The listing builds one solid part. Answer for the finished solid, in the listing's coordinates (mm). Face numbers are marked on the shaded views. A direction names the side the tool comes from. Give positions to 0.01 mm unless a question says otherwise; leave off trailing zeros. Write each loop counter-clockwise with the first axis right and the second up, starting at its lowest first coordinate (ties: lowest second). Pieces come first, ordered by that corner, then holes. Notation, with made-up numbers: (81.25, 49) - (89.25, 49) arc R21 cw to (89.25, 76) - close; hole circle Ø5 at (35.25, 86). An arc over 180 degrees is marked (long way). Return JSON: item names as keys, results as strings.
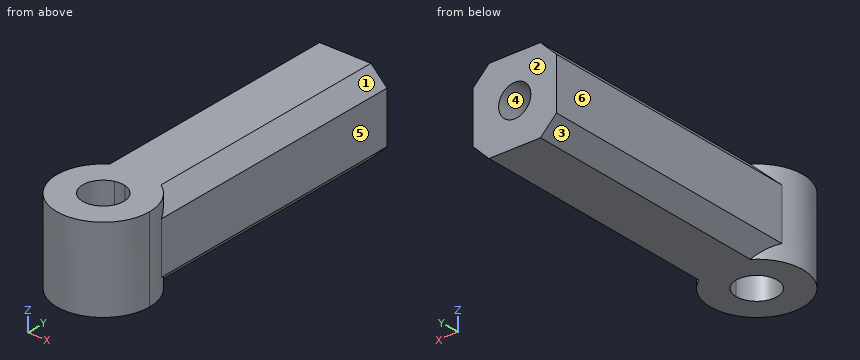
from build123d import *

# Parameters (mm, degrees)
F3_DEPTH = 6.5
F4_SIZE  = 1.25
F5_R     = 1.25
F6_DEPTH = 20


with BuildPart() as f3:
    # F2 (on Top) → F3 (new body)
    with BuildSketch(Plane.XY):
        with BuildLine():
            ThreePointArc((-3.25, 1.5483862567), (0, 3.6), (3.25, 1.5483862567))
            Line((3.25, 1.5483862567), (3.25, 22.5483862567))
            Line((3.25, 22.5483862567), (-3.25, 22.5483862567))
            Line((-3.25, 22.5483862567), (-3.25, 1.5483862567))
        make_face()
        with BuildLine():
            ThreePointArc((-0.4031128874, 1.5483862567), (0, 1.6), (0.4031128874, 1.5483862567))
            Line((0.4031128874, 1.5483862567), (3.25, 1.5483862567))
            ThreePointArc((3.25, 1.5483862567), (0, 3.6), (-3.25, 1.5483862567))
            Line((-3.25, 1.5483862567), (-0.4031128874, 1.5483862567))
        make_face()
        with BuildLine():
            ThreePointArc((0.4031128874, 1.5483862567), (1.2658950628, 0.9785242409), (1.6, 0))
            ThreePointArc((1.6, 0), (-0.9785242409, -1.2658950628), (-0.4031128874, 1.5483862567))
            Line((-0.4031128874, 1.5483862567), (-3.25, 1.5483862567))
            ThreePointArc((-3.25, 1.5483862567), (-0.7937253933, -3.5114099732), (3.6, 0))
            ThreePointArc((3.6, 0), (3.5114099732, 0.7937253933), (3.25, 1.5483862567))
            Line((3.25, 1.5483862567), (0.4031128874, 1.5483862567))
        make_face()
    extrude(amount=F3_DEPTH)

    # F4
    f4_edges = [f3.edges().sort_by_distance(p)[0] for p in [
        (3.25, 12.048386, 6.5),
        (-3.25, 12.048386, 6.5),
        (3.25, 12.048386, 0),
        (-3.25, 12.048386, 0),
    ]]
    chamfer(f4_edges, length=F4_SIZE)

    # F5 (on face) → F6 (cut)
    with BuildSketch(Plane(origin=(0, 22.5483862567, 0), x_dir=(-1, 0, 0), z_dir=(0, 1, 0))):
        with Locations((0, 3.25)):
            Circle(F5_R)
    extrude(amount=-F6_DEPTH, mode=Mode.SUBTRACT)


solid = f3.part
Item 1: Consider L1, parallel to Z at x = 0, y = 10; L2, parallel to Y at x = 0, z = 1.5; L3, parallel to Y at x = 0, z = 3.25. Determine where each line is inside the solid, lowest interval first.
Answer below:
{"L1": "z = 0 to 2, 4.5 to 6.5", "L2": "y = -3.6 to -1.6, 1.6 to 22.55", "L3": "y = -3.6 to -1.6, 1.6 to 2.55"}
Item 2: Flat-ended cylindrical pins translate along their axes: P1, Ø1, axis at y = -1, z = 3.5, coming from the -X side; P2, Ø1.2, axis at y = 17, z = 2.5, coming from the -X side; P3, Ø2, axis at x = -1.5, z = 3, coming from the -Y side. Find the tip coordinate at first contact, or state that the pin passes through.
Answer below:
{"P1": "stops at x = -3.57", "P2": "stops at x = -3.25", "P3": "stops at y = -3.57"}
Item 3: For the marked faces 1, 2 and 3, determine the directions among +Z, -Z, +X, -X, +Y, -Y from which every point of the face is accessible in a straight line to the end or side of a thin tool.
Answer below:
{"face 1": "+Z, +X, +Y", "face 2": "+Z, -Z, +X, -X, +Y", "face 3": "-Z, -X, +Y"}
Item 4: A cutting plane is placed at B-B on z = 3.25. Determine the outline of the cut face in (x, y), then the cut area to 3 significant figures.
Answer below:
{"outline": "(-3.25, 1.55) arc R3.6 ccw (long way) to (3.25, 1.55) - (3.25, 22.55) - (1.25, 22.55) - (1.25, 2.55) - (-1.25, 2.55) - (-1.25, 22.55) - (-3.25, 22.55) - close; hole circle Ø3.2 at (0, 0)", "area": "110 mm²"}
Item 5: The mould has two halves that part along X. Classify the marked faces 4, 5 and 6: +X half, -X half, draft (parallel to the pull), parting line (faces both ways), or undercut.
Answer below:
{"face 4": "undercut", "face 5": "+X half", "face 6": "-X half"}
Item 6: A cutting plane is placed at C-C on y = 6. Determine the outline of the cut face in (x, z), then the cut area to 3 significant figures.
Answer below:
{"outline": "(-3.25, 1.25) - (-2, 0) - (2, 0) - (3.25, 1.25) - (3.25, 5.25) - (2, 6.5) - (-2, 6.5) - (-3.25, 5.25) - close; hole circle Ø2.5 at (0, 3.25)", "area": "34.2 mm²"}
Item 7: A cutting plane is placed at A-A on x = 0. Determine the outline of the cut face in (y, z).
Answer below:
{"outline": "(-3.6, 0) - (-1.6, 0) - (-1.6, 6.5) - (-3.6, 6.5) - close; (1.6, 0) - (22.55, 0) - (22.55, 2) - (2.55, 2) - (2.55, 4.5) - (22.55, 4.5) - (22.55, 6.5) - (1.6, 6.5) - close"}
Item 8: A cutting plane is placed at D-D on x = -3. Determine the outline of the cut face in (y, z).
Answer below:
{"outline": "(-1.99, 0) - (1.99, 0) - (1.99, 1) - (22.55, 1) - (22.55, 5.5) - (1.99, 5.5) - (1.99, 6.5) - (-1.99, 6.5) - close"}
